from build123d import *

# Parameters (mm, degrees)
F0_R     = 1.625
F1_DEPTH = 2.5
F2_R     = 1.4
F3_DEPTH = 2.501
F4_R     = 1.5


with BuildPart() as f1:
    # F0 (on Front) → F1 (new body)
    with BuildSketch(Plane.XZ):
        with BuildLine():
            ThreePointArc((0, 4), (1.171573, 1.171573), (4, 0))
            Line((4, 0), (36.33, 0))
            ThreePointArc((36.33, 0), (39.158427, 1.171573), (40.33, 4))
            Line((40.33, 4), (40.33, 36.2))
            ThreePointArc((40.33, 36.2), (39.158427, 39.028427), (36.33, 40.2))
            Line((36.33, 40.2), (4, 40.2))
            ThreePointArc((4, 40.2), (1.171573, 39.028427), (0, 36.2))
            Line((0, 36.2), (0, 4))
        make_face()
        with Locations((4.125, 4.125)):
            Circle(F0_R, mode=Mode.SUBTRACT)
        with Locations((36.205, 4.125)):
            Circle(F0_R, mode=Mode.SUBTRACT)
        with Locations((4.125, 36.075)):
            Circle(F0_R, mode=Mode.SUBTRACT)
        with Locations((36.205, 36.075)):
            Circle(F0_R, mode=Mode.SUBTRACT)
    extrude(amount=F1_DEPTH)

    # F2 (on face) → F3 (cut, through all)
    with BuildSketch(Plane.XZ.offset(2.5)):
        with Locations((8.33, 31.83)):
            Circle(F2_R)
        with Locations((32, 31.83)):
            Circle(F2_R)
        with Locations((32, 8.37)):
            Circle(F2_R)
        with Locations((8.33, 8.37)):
            Circle(F2_R)
        with BuildLine():
            ThreePointArc((8.33, 19.415), (20.165, 8.37), (32, 19.415))
            Line((32, 19.415), (8.33, 19.415))
        make_face()
        with BuildLine():
            Line((8.33, 20.785), (32, 20.785))
            ThreePointArc((32, 20.785), (20.165, 31.83), (8.33, 20.785))
        make_face()
    extrude(amount=-F3_DEPTH, mode=Mode.SUBTRACT)

    # F4
    f4_edges = [f1.edges().sort_by_distance(p)[0] for p in [
        (8.33, -1.25, 20.785),
        (32, -1.25, 20.785),
        (32, -1.25, 19.415),
        (8.33, -1.25, 19.415),
    ]]
    fillet(f4_edges, radius=F4_R)


solid = f1.part
For this review, take the finished solid that the model builds, in its own axes (mm). A direction names the side the tool comes from. Round coordinates to 2 decimals unless told otherwise and drop trailing zeros. Write each loop counter-clockwise with the first axis right and the second up, starting at its lowest first coordinate (ties: lowest second). Pieces come first, ordered by that corner, then holes. Notation, with made-up numbers: (41, 72) -> (58, 72) arc R24 ccw to (58, 97) -> close; hole circle Ø2 at (52, 29). An arc over 180 degrees is marked (long way). Put each result on its own line as item: value.
Q1. To check wall thickness, follow L1, parallel to Z at x = 32, y = -1.75; L2, parallel to Z at x = 22.5, y = -1.4 (3 decimals); L3, parallel to X at y = -2.15, z = 4.5. State the ranges of each line that lie inside material, in increasing order. Write a range as [from, to].
Determined:
L1: z = [0, 6.97], [9.77, 30.43], [33.23, 40.2]
L2: z = [0, 8.602], [19.415, 20.785], [31.598, 40.2]
L3: x = [0, 2.54], [5.71, 34.62], [37.79, 40.33]
Q2. Consider section A-A on z = 37. State the section outline as (x, y) points.
Determined:
outline: (0.08, -2.5) -> (2.79, -2.5) -> (2.79, 0) -> (0.08, 0) -> close; (5.46, -2.5) -> (34.87, -2.5) -> (34.87, 0) -> (5.46, 0) -> close; (37.54, -2.5) -> (40.25, -2.5) -> (40.25, 0) -> (37.54, 0) -> close
Q3. Consider section B-B on y = -0.65. Give the number of separate pieces and of enclosed holes in the cut face, and give its area (3 significant figures).
Determined:
separate pieces: 1
enclosed holes: 10
area: 1,150 mm^2
Q4. The part is to be moulded in two halves that separate along Z. For faces 3 (the flat face through (20, 0, 20)), 4 (the flat face through (20, -1, 0)), 5 (the cylindrical face through (8.027, -1.268, 7.003)), say which applies: released by +Z, released by -Z, zero draft, split by the parting line, or undercut.
Determined:
face 3: zero draft
face 4: released by -Z
face 5: undercut
Q5. Machinability: for faces 1 (the cylindrical face through (20.388, -1.268, 31.828)), 2 (the flat face through (20, -1, 40.2)), which of the approach directions +Z, -Z, +X, -X, +Y, -Y give a long, thin tool a straight path to every point of the face, cutting with its end or side? Answer none if there is none.
Determined:
face 1: +Y, -Y
face 2: +Z, +X, -X, +Y, -Y
Q6. Clearance check with a flat-ended pin moving along its axis: pin 1 Ø1.9 at (x, z) = (36.205, 4.125) entering from +Y. State where the tip first meets the part, or that it passes through.
Determined:
pin 1: passes through
Q7. Consider section D-D on z = 17. State the section outline as (x, y) points.
Determined:
outline: (0, -2.5) -> (8.75, -2.5) -> (8.75, 0) -> (0, 0) -> close; (31.58, -2.5) -> (40.33, -2.5) -> (40.33, 0) -> (31.58, 0) -> close
Q8. Consider section C-C on x = 25.5. State the section outline as (y, z) points (3 decimals), and give its area (3 significant figures).
Determined:
outline: (-2.5, 0) -> (0, 0) -> (0, 9.637) -> (-2.5, 9.637) -> close; (-2.5, 19.415) -> (0, 19.415) -> (0, 20.785) -> (-2.5, 20.785) -> close; (-2.5, 30.563) -> (0, 30.563) -> (0, 40.2) -> (-2.5, 40.2) -> close
area: 51.6 mm^2
